```python
from build123d import *

# Parameters (mm, degrees)
SKETCH1_W                      = 6.35
SKETCH1_H                      = 9.525
BOSS_EXTRUDE1_DEPTH            = 38.1
F_8_32_TAPPED_HOLE1_AT_2_COUNT = 2
F_8_32_TAPPED_HOLE1_AT_2_PITCH = 63.5
F_8_32_TAPPED_HOLE2_AT_2_COUNT = 2
F_8_32_TAPPED_HOLE2_AT_2_PITCH = 50.8


with BuildPart() as part:
    # Sketch1 → Boss-Extrude1 (new, symmetric)
    with BuildSketch(Plane(origin=(0, 0, 0), x_dir=(0, 0, -1), z_dir=(1, 0, 0))):
        Rectangle(SKETCH1_W, SKETCH1_H)
    extrude(amount=BOSS_EXTRUDE1_DEPTH, both=True)

    # Sketch2 → #8-32 Tapped Hole1 (revolve, cut)
    with BuildSketch(Plane(origin=(31.75, 4.7625, 0), x_dir=(0, 0, 1), z_dir=(1, 0, 0))):
        Polygon((0, 0), (0, 9.525), (2.286, 9.525), (1.7272, 8.9662), (1.7272, 0.5588), (2.286, 0), align=None)
    f_8_32_tapped_hole1 = revolve(axis=Axis((31.75, 11.1125, 0), (0, -1, 0)), mode=Mode.SUBTRACT)

    # #8-32 Tapped Hole1 at 2: #8-32 Tapped Hole1 ×2
    with Locations(*[(-i * F_8_32_TAPPED_HOLE1_AT_2_PITCH, 0, 0) for i in range(1, F_8_32_TAPPED_HOLE1_AT_2_COUNT)]):
        add(f_8_32_tapped_hole1, mode=Mode.SUBTRACT)

    # Sketch4 → #8-32 Tapped Hole2 (revolve, cut)
    with BuildSketch(Plane(origin=(25.4, -1.5875, 3.175), x_dir=(0, -1, 0), z_dir=(1, 0, 0))):
        Polygon((0, 0), (0, 6.35), (2.286, 6.35), (1.7272, 5.7912), (1.7272, 0.5588), (2.286, 0), align=None)
    f_8_32_tapped_hole2 = revolve(axis=Axis((25.4, -1.5875, 9.525), (0, 0, -1)), mode=Mode.SUBTRACT)

    # #8-32 Tapped Hole2 at 2: #8-32 Tapped Hole2 ×2
    with Locations(*[(-i * F_8_32_TAPPED_HOLE2_AT_2_PITCH, 0, 0) for i in range(1, F_8_32_TAPPED_HOLE2_AT_2_COUNT)]):
        add(f_8_32_tapped_hole2, mode=Mode.SUBTRACT)


solid = part.part
```
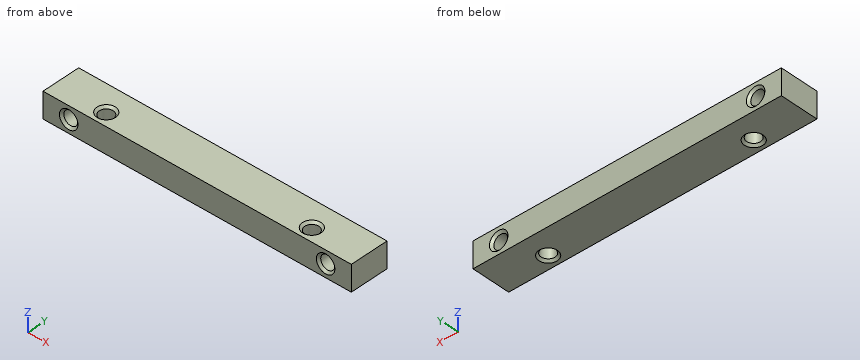
The listing builds one solid part. Answer for the finished solid, in the listing's coordinates (mm). Coordinates: 2 decimals unless noted, no trailing zeros. Write each loop counter-clockwise with the first axis right and the second up, starting at its lowest first coordinate (ties: lowest second). Pieces come first, ordered by that corner, then holes. Notation, with made-up numbers: (52, 55) - (63, 55) arc R25 ccw to (63, 94) - close; hole circle Ø1 at (64, 60.25). An arc over 180 degrees is marked (long way). One line per item, written item: value.
1) Consider line 1 along X through (y, z) = (0.5, 0); line 2 along X through (y, z) = (-1.75, 0); line 3 along Y through (x, z) = (-25.4, 0.3). Determine where each line is inside the solid, lowest interval first. Write a range as from..to.
Geometry check:
line 1: x = -38.1..-33.48, -30.02..30.02, 33.48..38.1
line 2: x = -38.1..-33.48, -30.02..-27.12, -23.68..23.68, 27.12..30.02, 33.48..38.1
line 3: y = -4.76..-3.31, 0.14..4.76
2) Find section B-B (x = -31.75). Give the vertices of the cut face in (y, z) (1 decimal).
Geometry check:
outline: (-4.8, -3.2) - (4.8, -3.2) - (4.8, -2.3) - (4.2, -1.7) - (-4.2, -1.7) - (-4.8, -2.3) - close; (-4.8, 2.3) - (-4.2, 1.7) - (4.2, 1.7) - (4.8, 2.3) - (4.8, 3.2) - (-4.8, 3.2) - close
3) Each of these flat-tipped pins is pushed along its axis until it touches: pin 1 Ø2 at (x, y) = (25.4, -1.59) entering from -Z; pin 2 Ø4 at (x, y) = (-25.4, -1.59) entering from -Z. Where does it stop, or does it pass through?
Geometry check:
pin 1: passes through
pin 2: stops at z = -2.89
4) Find section A-A (z = 0). Give the vertices of the cut face in (x, y), and give its area (3 significant figures).
Geometry check:
outline: (-38.1, -4.76) - (-34.04, -4.76) - (-33.48, -4.2) - (-33.48, 4.2) - (-34.04, 4.76) - (-38.1, 4.76) - close; (-30.02, -4.2) - (-29.46, -4.76) - (29.46, -4.76) - (30.02, -4.2) - (30.02, 4.2) - (29.46, 4.76) - (-29.46, 4.76) - (-30.02, 4.2) - close; (33.48, -4.2) - (34.04, -4.76) - (38.1, -4.76) - (38.1, 4.76) - (34.04, 4.76) - (33.48, 4.2) - close; hole circle Ø3.45 at (-25.4, -1.59); hole circle Ø3.45 at (25.4, -1.59)
area: 640 mm2
5) Find section C-C (y = -1.5). Count the separate pieces of the cut face and the enclosed holes in it, and give its area (3 significant figures).
Geometry check:
separate pieces: 3
enclosed holes: 2
area: 420 mm2
